from build123d import *

# Parameters (mm, degrees)
F1_DEPTH = 4.7625


# Not quite as in the source:
# - ends of sketch curves that miss each other by under 0.0002 mm in the source are joined


with BuildPart() as f1:
    # F0 (on Right) → F1 (new body)
    with BuildSketch(Plane.YZ):
        with BuildLine():
            ThreePointArc((-10.3035716562, 255.2451451351), (-14.739191866, 253.5576398603), (-19.1058595605, 255.4162990395))
            Line((-19.1058595605, 255.4162990395), (-19.2069466, 255.517396))
            Line((-19.2069466, 255.517396), (-46.1477106, 282.45816))
            ThreePointArc((-46.1477106, 282.45816), (-50.6378374197, 284.3180242), (-55.1279617605, 282.4581649605))
            Line((-55.1279617605, 282.4581649605), (-303.1270036, 34.4591132))
            ThreePointArc((-303.1270036, 34.4591132), (-304.9868678, 29.9689938197), (-303.1269958605, 25.4788747395))
            Line((-303.1269958605, 25.4788747395), (-271.6961038, -5.9520328))
            Line((-271.6961038, -5.9520328), (-10.3035716562, 255.2451451351))
        make_face()
    extrude(amount=F1_DEPTH)


solid = f1.part
Could you check a few things on this model? Use its own coordinates, in mm. Give positions to 0.01 mm unless a question says otherwise; leave off trailing zeros. Order: outer loops, then holes, each group sorted by start corner. A loop starts at its lowest first (then second) coordinate and runs counter-clockwise, first axis right, second up. Notation, with made-up numbers: (23, 14.5) -> (63, 14.5) arc R14 cw to (63, 22.5) -> close; hole circle Ø11 at (-5.5, 56.25). An arc over 180 degrees is marked (long way). Return JSON: item names as keys, results as strings.
1. For pin 1 Ø2 at (x, y) = (4, -261) entering from -Z; pin 2 Ø2 at (x, z) = (2.5, 114.5) entering from +Y, each with a flat end and sliding along its axis, tell me the tip position at first contact or that it passes through.
Answer list:
{"pin 1": "stops at z = 3.74", "pin 2": "stops at y = -150.15"}
2. Imagine slicing it at A-A on x = 3.15. List the corners of the cut face in (y, z) for me.
Answer list:
{"outline": "(-303.13, 25.48) -> (-271.7, -5.95) -> (-10.3, 255.25) arc R6.35 cw to (-19.11, 255.42) -> (-19.21, 255.52) -> (-46.15, 282.46) arc R6.35 ccw to (-55.13, 282.46) -> (-303.13, 34.46) arc R6.35 ccw to start"}
3. Imagine slicing it at C-C on z = 91.5. List the corners of the cut face in (x, y) for me.
Answer list:
{"outline": "(0, -246.09) -> (4.76, -246.09) -> (4.76, -174.17) -> (0, -174.17) -> close"}
4. I need wall thicknesses on line 1 (Z direction, x = 0.9, y = -291); line 2 (Y direction, x = 4, z = 123); line 3 (Y direction, x = 4.25, z = 95). Which ranges of each line are inside material? Lowest first, please. Write a range as from..to.
Answer list:
{"line 1": "z = 13.35..46.59", "line 2": "y = -214.59..-142.65", "line 3": "y = -242.59..-170.67"}
5. Imagine slicing it at B-B on y = -96. List the corners of the cut face in (x, z) for me.
Answer list:
{"outline": "(0, 169.61) -> (4.76, 169.61) -> (4.76, 241.59) -> (0, 241.59) -> close"}
